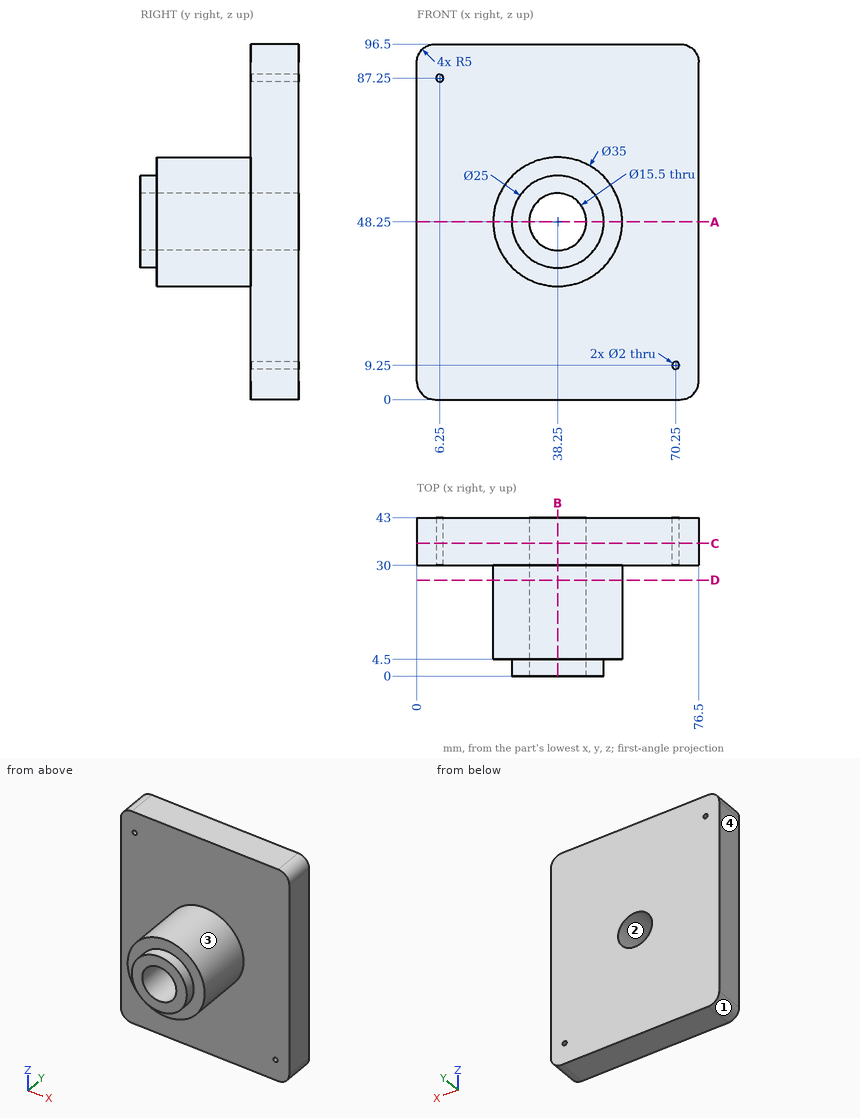
Could you check a few things on this drawing? It's one solid part, dimensions in mm from its lowest x, y, z. Coordinates: 2 decimals unless noted, no trailing zeros. Order: outer loops, then holes, each group sorted by start corner. A loop starts at its lowest first (then second) coordinate and runs counter-clockwise, first axis right, second up. Notation, with made-up numbers: (66, 41) - (97, 41) arc R18 cw to (97, 51) - close; hole circle Ø1 at (11, -30). An arc over 180 degrees is marked (long way). Answer as a JSON object with one key per item and string values. Group by question number.
Q1. Imagine slicing it at D-D (y = 26). Please give me the cut outline in (x, z), and give its area (3 significant figures).
Q2. Imagine slicing it at C-C (y = 36). Please give me the cut outline in (x, z), and give its area (3 significant figures).
Q3. Will these pins go through, and if not, where does the flat tip stop? P1, Ø6, axis at x = 27, z = 70.5, coming from the -Y side; P2, Ø6, axis at y = 16.5, z = 30, coming from the +X side; P3, Ø1, axis at x = 22.5, y = 12, coming from the -Z side.
Q4. We'd pull the mould along Z, two halves only. Please class the marked faces 1, 2, 3 and 4: +Z half, -Z half, draft (parallel to the pull), parting line (faces both ways), or undercut.
Q5. Imagine slicing it at B-B (x = 38.25). Please give me the cut outline in (y, z).
Q6. Imagine slicing it at A-A (z = 48.25). Please give me the cut outline in (x, y), and give its area (3 significant figures).
Q7. I need wall thicknesses on line 1 (Z direction, x = 38, y = 17); line 2 (X direction, y = 23, z = 48); line 3 (Z direction, x = 70.25, y = 34). Which ranges of each line are inside material? Lowest first, please. Write a range as from..to.
Determined:
{
 "1": {"outline": "circle Ø35 at (38.25, 48.25); hole circle Ø15.5 at (38.25, 48.25)", "area": "773 mm2"},
 "2": {"outline": "(0, 5) arc R5 ccw to (5, 0) - (71.5, 0) arc R5 ccw to (76.5, 5) - (76.5, 91.5) arc R5 ccw to (71.5, 96.5) - (5, 96.5) arc R5 ccw to (0, 91.5) - close; hole circle Ø2 at (6.25, 87.25); hole circle Ø15.5 at (38.25, 48.25); hole circle Ø2 at (70.25, 9.25)", "area": "7,170 mm2"},
 "3": {"P1": "stops at y = 30", "P2": "stops at x = 46.83", "P3": "stops at z = 39.67"},
 "4": {"face 1": "-Z half", "face 2": "undercut", "face 3": "parting line", "face 4": "draft"},
 "5": {"outline": "(0, 35.75) - (4.5, 35.75) - (4.5, 30.75) - (30, 30.75) - (30, 0) - (43, 0) - (43, 40.5) - (0, 40.5) - close; (0, 56) - (43, 56) - (43, 96.5) - (30, 96.5) - (30, 65.75) - (4.5, 65.75) - (4.5, 60.75) - (0, 60.75) - close"},
 "6": {"outline": "(0, 30) - (20.75, 30) - (20.75, 4.5) - (25.75, 4.5) - (25.75, 0) - (30.5, 0) - (30.5, 43) - (0, 43) - close; (46, 0) - (50.75, 0) - (50.75, 4.5) - (55.75, 4.5) - (55.75, 30) - (76.5, 30) - (76.5, 43) - (46, 43) - close", "area": "1,330 mm2"},
 "7": {"line 1": "z = 30.75..40.5, 56..65.75", "line 2": "x = 20.75..30.5, 46..55.75", "line 3": "z = 0..8.25, 10.25..96.5"}
}
